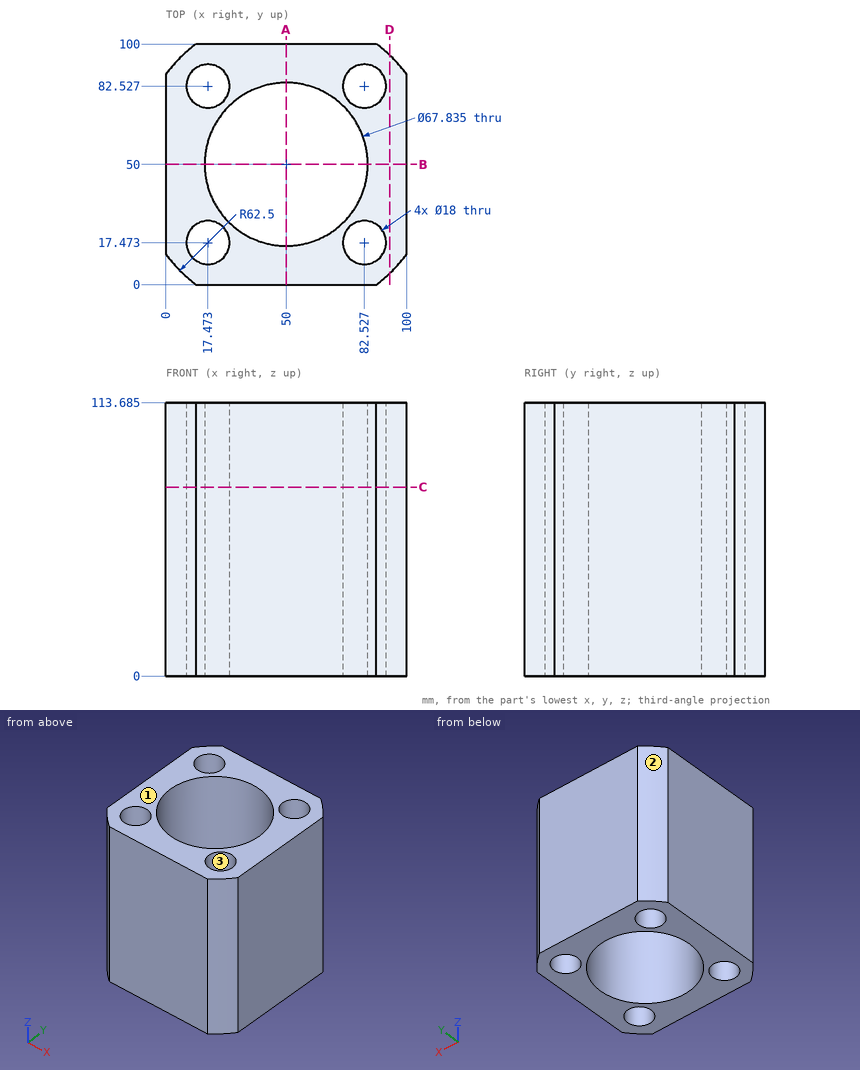
The drawing under review shows one solid part. Ordinate dimensions are in mm from its lowest x, y, z. Round coordinates to 2 decimals unless told otherwise and drop trailing zeros. Write each loop counter-clockwise with the first axis right and the second up, starting at its lowest first coordinate (ties: lowest second). Pieces come first, ordered by that corner, then holes.
(1) We need section A-A on x = 50. Give the boundary of the cut face in (y, z) (1 decimal), and give its area (3 significant figures).
(2) We need section D-D on x = 93. Give the boundary of the cut face in (y, z) (1 decimal), and give its area (3 significant figures).
(3) Insertion check: pin 1 (14.5 mm diameter, centred on x = 17.47, y = 17.47, fed in from +Z). The pin has a flat end and moves straight along its axis. Give the tip position at first contact, or say it passes through.
(4) Wall thickness on L1, parallel to Y at x = 49.5, z = 38.5; L2, parallel to X at y = 15.5, z = 107.5 (1 decimal); L3, parallel to X at y = 86, z = 94 (1 decimal): over which ranges is each line inside the solid? List them lowest first.
(5) Mouldability with a two-part tool opening along X and no side actions: class the marked faces 1, 2 and 3 as +X half, -X half, draft (parallel to the pull), parting line (faces both ways), or undercut.
(6) We need section C-C on z = 78.5. Give the boundary of the cut face in (x, y) (1 decimal).
Findings below:
1. outline: (0, 0) - (16.1, 0) - (16.1, 113.7) - (0, 113.7) - close; (83.9, 0) - (100, 0) - (100, 113.7) - (83.9, 113.7) - close
1. area: 3,660 mm2
2. outline: (4.6, 0) - (95.4, 0) - (95.4, 113.7) - (4.6, 113.7) - close
2. area: 10,300 mm2
3. pin 1: passes through
4. L1: y = 0 to 16.09, 83.91 to 100
4. L2: x = 0 to 8.7, 26.3 to 73.7, 91.3 to 100
4. L3: x = 0 to 9.2, 25.8 to 74.2, 90.8 to 100
5. face 1: draft
5. face 2: -X half
5. face 3: undercut
6. outline: (0, 12.5) arc R62.5 ccw to (12.5, 0) - (87.5, 0) arc R62.5 ccw to (100, 12.5) - (100, 87.5) arc R62.5 ccw to (87.5, 100) - (12.5, 100) arc R62.5 ccw to (0, 87.5) - close; hole circle Ø18 at (17.5, 17.5); hole circle Ø18 at (17.5, 82.5); hole circle Ø67.8 at (50, 50); hole circle Ø18 at (82.5, 17.5); hole circle Ø18 at (82.5, 82.5)
